Can you work these out from the model? Positions are in its coordinate system, mm. A direction names the side the tool comes from. Give positions to 0.01 mm unless a question says otherwise; leave off trailing zeros. Write each loop counter-clockwise with the first axis right and the second up, starting at its lowest first coordinate (ties: lowest second). Pieces come first, ordered by that corner, then holes.
1. Thinking about a two-plate mould opening in Y: for faces 1 (the cylindrical face through (151.863, 8.085, 7.692)), 2 (the flat face through (79, 6, 0)), 3 (the flat face through (143, 5.25, 0)), which applies, pulls with the +Y half, pulls with the -Y half, needs draft (parallel to the pull), parting line crosses it, or undercut?
2. Suppose I cut it at C-C (x = 28). Please give me the cut outline in (y, z).
3. I'm going to push flat-ended pins straight in: pin 1 (21 mm diameter, centred on x = 134, y = -0.5, fed in from +Z); pin 2 (13 mm diameter, centred on x = 79, z = -1, fed in from +Y); pin 3 (21 mm diameter, centred on x = 134.5, y = 5, fed in from -Z); pin 4 (5 mm diameter, centred on x = 51.5, y = 10, fed in from -Z). Where does each tip first touch, or does it pass through?
4. If I drill on probe 1 along X at (y, z) = (8, 0); probe 2 along Z at (x, y) = (130, 1); probe 3 along X at (y, z) = (40, -19), over which ranges is the centre line in solid material (lowest first)?
5. Suppose I cut it at B-B (y = -3). Please give me the cut outline in (x, z), and give its area (3 significant figures).
6. Suppose I cut it at A-A (x = 137). Please give me the cut outline in (y, z).
7. Suppose I cut it at D-D (z = 20). Please give me the cut outline in (x, y).
8. On a 3-axis mill with a long thin cutter (end or side, diameter ignored), from which of +Z, -Z, +X, -X, +Y, -Y can I reach the whole of each face in a straight line? I mean faces 4 (the flat face through (131, 0, 0)), 5 (the flat face through (140, 11, 0)), 6 (the flat face through (44, 5, -5.8)). Say none if no direction works.
Autodesk Inventor part; units mm, degrees
ref_plane "YZ Plane" through (0, 0, 0) normal (1, 0, 0) x (0, 1, 0)
ref_plane "XZ Plane" through (0, 0, 0) normal (0, 1, 0) x (-1, 0, 0)
ref_plane "XY Plane" through (0, 0, 0) normal (0, 0, 1) x (1, 0, 0)
sketch "草圖1" plane through (0, 0, 0) normal (1, 0, 0) x (0, 1, 0)
  line L0 (6, 5.8) -> (-6, 5.8)
  line L1 (-6, 5.8) -> (-6, -5.8)
  line L2 (-6, -5.8) -> (6, -5.8)
  line L3 (6, -5.8) -> (6, 5.8)
  line L4 (6, 5.8) -> (-6, -5.8) construction
  line L5 (-6, 5.8) -> (6, -5.8) construction
  point P0 (0, 0)
  dimension "d2" = 12
  dimension "d3" = 11.6
extrude "擠出1" add sketch "草圖1" along normal blind 125
sketch "草圖2" plane through (0, 6, 5.8) normal (0, 1, 0) x (1, 0, 0)
  line L0 (0, 0) -> (125, 0)
  line L1 (0, 11.6) -> (125, 11.6)
  line L2 (0, 0) -> (25, 0)
  line L3 (25, 0) -> (25, 11.6)
  line L4 (25, 11.6) -> (0, 11.6)
  line L5 (0, 11.6) -> (0, 0)
  point P0 (0, 5.8)
  point P1 (0, 11.6)
  dimension "d6" = 25
extrude "擠出2" add sketch "草圖2" along normal blind 30.5
sketch "草圖3" plane through (0, 36.5, 5.8) normal (0, 1, 0) x (1, 0, 0)
  line L0 (25, 35.8) -> (0, 35.8)
  line L1 (0, 35.8) -> (0, -23.8)
  line L2 (0, -23.8) -> (25, -23.8)
  line L3 (25, -23.8) -> (25, 35.8)
  line L4 (25, 0) -> (25, 11.6)
  line L5 (25, 0) -> (125, 0)
  point P0 (0, 5.8)
  point P1 (25, 5.8)
  dimension "d9" = 25
  dimension "d10" = 59.6
  dimension "d11" = 23.8
extrude "擠出3" add sketch "草圖3" along normal blind 11.6
sketch "草圖4" plane through (125, 0, 0) normal (1, 0, 0) x (0, 0, -1)
  line L0 (-11, -11) -> (11, -11)
  line L1 (11, -11) -> (11, 11)
  line L2 (11, 11) -> (-11, 11)
  line L3 (-11, 11) -> (-11, -11)
  line L4 (-11, -11) -> (11, 11) construction
  line L5 (11, -11) -> (-11, 11) construction
  point P0 (0, 0)
  dimension "d14" = 22
  dimension "d15" = 22
extrude "擠出4" add sketch "草圖4" along normal blind 30
sketch "草圖5" plane through (125, -11, -11) normal (0, 0, -1) x (-1, 0, 0)
  line L0 (-30, 0) -> (-30, 22)
  line L1 (-30, 5.75) -> (-6, 5.75)
  line L2 (-6, 5.75) -> (-6, 16.25)
  line L3 (-6, 16.25) -> (-30, 16.25)
  line L4 (-30, 16.25) -> (-30, 5.75)
  line L5 (0, 17) -> (0, 5)
  line L6 (0, 11) -> (-32.9331, 11) construction
  point P0 (125, 11)
  dimension "d18" = 10.5
  dimension "d19" = 24
extrude "擠出5" cut sketch "草圖5" against normal blind 30
sketch "草圖6" plane through (125, 11, 11) normal (0, 1, 0) x (1, 0, 0)
  line L0 (6, 22) -> (6, 0) construction
  line L1 (6, 22) -> (6, 0) construction
  line L2 (6, 11) -> (33.0459, 11) construction
  circle A0 centre (21, 11) radius 1.6
  point P0 (-125, 11)
  dimension "d22" = 15
  dimension "d23" = 3.2
extrude "擠出6" cut sketch "草圖6" against normal blind 30
fillet "圓角1" radius 11 4 edges at (155, 8.125, -11) (155, 8.125, 11) (155, -8.125, 11) (155, -8.125, -11)
fillet "圓角2" radius 10 4 edges at (125, 6, 0) (125, 0, 5.8) (125, 0, -5.8) (125, -6, 0)
chamfer "倒角1" distance 15 angle 45 1 edges at (25, 6, 0)
fillet "圓角3" radius 2 4 edges at (12.5, 48.1, -30) (12.5, 36.5, -30) (12.5, 36.5, 29.6) (12.5, 48.1, 29.6)
fillet "圓角4" radius 1 2 edges at (12.5, 36.5, 5.8) (12.5, 36.5, -5.8)
properties part number "support"
Checks:
1. face 1: needs draft
1. face 2: pulls with the +Y half
1. face 3: undercut
2. outline: (-6, -5.8) - (18, -5.8) - (18, 5.8) - (-6, 5.8) - close
3. pin 1: stops at z = 11
3. pin 2: stops at y = 6
3. pin 3: stops at z = -11
3. pin 4: passes through
4. probe 1: x = 0 to 38, 122.34 to 144.4, 147.6 to 155
4. probe 2: z = -11 to 11
4. probe 3: x = 0 to 25
5. outline: (0, -5.8) - (116.23, -5.8) arc R10 cw to (125, -11) - (131, -11) - (131, 11) - (125, 11) arc R10 cw to (116.23, 5.8) - (0, 5.8) - close
5. area: 1,610 mm2
6. outline: (-11, -11) - (-5.25, -11) - (-5.25, 11) - (-11, 11) - close; (5.25, -11) - (11, -11) - (11, 11) - (5.25, 11) - close
7. outline: (0, 36.5) - (25, 36.5) - (25, 48.1) - (0, 48.1) - close
8. face 4: +Z, -Z, +X
8. face 5: +Z, -Z, +X, +Y
8. face 6: -Z, -X, -Y
